from build123d import *

# Parameters (mm, degrees)
MODEL_R             = 0.5
MODEL_R_2           = 0.75
BOSS_EXTRUDE1_DEPTH = 2


with BuildPart() as part:
    # Model → Boss-Extrude1 (new body)
    with BuildSketch(Plane.XY):
        with BuildLine():
            Line((2, 0), (18, 0))
            ThreePointArc((18, 0), (19.414213562, 0.585786438), (20, 2))
            Line((20, 2), (20, 5))
            Line((20, 5), (13.75, 5))
            Line((13.75, 5), (13.75, 7))
            Line((13.75, 7), (20, 7))
            Line((20, 7), (20, 38.2))
            ThreePointArc((20, 38.2), (18.535533906, 41.735533906), (15, 43.2))
            Line((15, 43.2), (5, 43.2))
            ThreePointArc((5, 43.2), (1.464466094, 41.735533906), (0, 38.2))
            Line((0, 38.2), (0, 7))
            Line((0, 7), (6.25, 7))
            Line((6.25, 7), (6.25, 5))
            Line((6.25, 5), (0, 5))
            Line((0, 5), (0, 2))
            ThreePointArc((0, 2), (0.585786438, 0.585786438), (2, 0))
        make_face()
        with Locations((3, 18)):
            Circle(MODEL_R, mode=Mode.SUBTRACT)
        with Locations((17, 18)):
            Circle(MODEL_R, mode=Mode.SUBTRACT)
        with Locations((14, 9.5)):
            Circle(MODEL_R_2, mode=Mode.SUBTRACT)
        with Locations((6, 9.5)):
            Circle(MODEL_R_2, mode=Mode.SUBTRACT)
        with Locations((17.25, 2.5)):
            Circle(MODEL_R_2, mode=Mode.SUBTRACT)
        with Locations((2.75, 2.5)):
            Circle(MODEL_R_2, mode=Mode.SUBTRACT)
    extrude(amount=BOSS_EXTRUDE1_DEPTH)


solid = part.part
Part model, mm, in its own coordinate system. A direction names the side the tool comes from. Coordinates: 2 decimals unless noted, no trailing zeros. Loops run counter-clockwise (first coordinate to the right, second up) from the corner with the lowest first, then second, coordinate; pieces in that order, holes last. Notation, with made-up numbers: M -21,-8.5 L 19,-8.5 A9 ccw 19,-4.5 Z; hole C 73,19 d6. An arc over 180 degrees is marked long. Use a Markdown table: item, result. Add a question column.
Q1. Cut at C-C (x = 17). Write the cut outline in (y, z).
Q2. Mould opens along Y. For faces 4 (the flat face through (6.25, 6, 1)), 5 (the flat face through (0, 23, 1)), 6 (the flat face through (10, 0, 1)) say: +Y half, -Y half, draft (parallel to the pull), parting line (faces both ways), or undercut.
Q3. Which spindle directions (+Z, -Z, +X, -X, +Y, -Y) get a long thin tool onto all of the face, cutting with end or side? Do faces 1 (the cylindrical face through (16.655, 2.044, 0.986)), 2 (the flat face through (3, 7, 1)), 3 (the flat face through (17, 5, 1)). Say none if no direction does.
Q4. Cut at A-A (y = 9.5). Write the cut outline in (x, z), and give its area (3 significant figures).
Q5. Pin check, flat tips, straight feed: P1, Ø1.2, axis at x = 14, y = 9.5, coming from the +Z side; P2, Ø0.6, axis at x = 1.5, z = 1, coming from the -Y side. Stop position of each tip, or through.
Q6. Cut at B-B (z = 1.35). Write the cut outline in (x, y).
Q7. Probe L1, parallel to Y at x = 6, z = 1.5; L2, parallel to X at y = 9, z = 0.85; L3, parallel to Y at x = 2.75, z = 1.35. List the from-to ranges inside material, lowest first.
Worked out:
| question | item | result |
|---|---|---|
| 1 | outline | M 0,0 L 1.79,0 L 1.79,2 L 0,2 Z; M 3.21,0 L 5,0 L 5,2 L 3.21,2 Z; M 7,0 L 17.5,0 L 17.5,2 L 7,2 Z; M 18.5,0 L 42.78,0 L 42.78,2 L 18.5,2 Z |
| 2 | face 4 | undercut |
| 2 | face 5 | draft |
| 2 | face 6 | -Y half |
| 3 | face 1 | +Z, -Z |
| 3 | face 2 | +Z, -Z, -X |
| 3 | face 3 | +Z, -Z, +X |
| 4 | outline | M 0,0 L 5.25,0 L 5.25,2 L 0,2 Z; M 6.75,0 L 13.25,0 L 13.25,2 L 6.75,2 Z; M 14.75,0 L 20,0 L 20,2 L 14.75,2 Z |
| 4 | area | 34.0 mm2 |
| 5 | P1 | passes through |
| 5 | P2 | stops at y = 0.01 |
| 6 | outline | M 0,2 A2 ccw 2,0 L 18,0 A2 ccw 20,2 L 20,5 L 13.75,5 L 13.75,7 L 20,7 L 20,38.2 A5 ccw 15,43.2 L 5,43.2 A5 ccw 0,38.2 L 0,7 L 6.25,7 L 6.25,5 L 0,5 Z; hole C 2.75,2.5 d1.5; hole C 3,18 d1; hole C 6,9.5 d1.5; hole C 14,9.5 d1.5; hole C 17.25,2.5 d1.5; hole C 17,18 d1 |
| 7 | L1 | y = 0 to 5, 7 to 8.75, 10.25 to 43.2 |
| 7 | L2 | x = 0 to 5.44, 6.56 to 13.44, 14.56 to 20 |
| 7 | L3 | y = 0 to 1.75, 3.25 to 5, 7 to 17.57, 18.43 to 42.67 |
